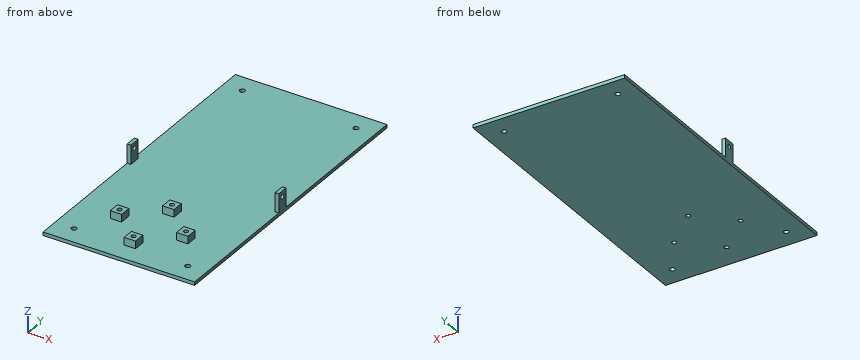
```python
from build123d import *

# Parameters (mm, degrees)
F0_R     = 7
F0_W     = 30
F0_H     = 30
F1_DEPTH = 9
F0_R_2   = 6
F2_DEPTH = 29
F0_W_2   = 10
F3_DEPTH = 59
F4_R     = 6
F5_DEPTH = 486


with BuildPart() as f1:
    # F0 (on Top) → F1 (new body)
    with BuildSketch(Plane.XY):
        Polygon((0, 350), (0, 0), (400, 0), (400, 350), (390, 350), (390, 380), (400, 380), (400, 800), (0, 800), (0, 380), (10, 380), (10, 350), align=None)
        with Locations((50, 50)):
            Circle(F0_R, mode=Mode.SUBTRACT)
        with Locations((197.5, 65)):
            Rectangle(F0_W, F0_H, mode=Mode.SUBTRACT)
        with Locations((110, 145)):
            Rectangle(F0_W, F0_H, mode=Mode.SUBTRACT)
        with Locations((197.5, 225)):
            Rectangle(F0_W, F0_H, mode=Mode.SUBTRACT)
        with Locations((285, 145)):
            Rectangle(F0_W, F0_H, mode=Mode.SUBTRACT)
        with Locations((350, 50)):
            Circle(F0_R, mode=Mode.SUBTRACT)
        with Locations((50, 750)):
            Circle(F0_R, mode=Mode.SUBTRACT)
        with Locations((350, 750)):
            Circle(F0_R, mode=Mode.SUBTRACT)
    extrude(amount=F1_DEPTH)

    # F0 (on Top) → F2 (join)
    with BuildSketch(Plane.XY):
        with Locations((110, 145)):
            Rectangle(F0_W, F0_H)
        with Locations((110, 145)):
            Circle(F0_R_2, mode=Mode.SUBTRACT)
        with Locations((197.5, 225)):
            Rectangle(F0_W, F0_H)
        with Locations((197.5, 225)):
            Circle(F0_R_2, mode=Mode.SUBTRACT)
        with Locations((197.5, 65)):
            Rectangle(F0_W, F0_H)
        with Locations((197.5, 65)):
            Circle(F0_R_2, mode=Mode.SUBTRACT)
        with Locations((285, 145)):
            Rectangle(F0_W, F0_H)
        with Locations((285, 145)):
            Circle(F0_R_2, mode=Mode.SUBTRACT)
    extrude(amount=F2_DEPTH)

    # F0 (on Top) → F3 (join)
    with BuildSketch(Plane.XY):
        with Locations((5, 365)):
            Rectangle(F0_W_2, F0_H)
        with Locations((395, 365)):
            Rectangle(F0_W_2, F0_H)
    extrude(amount=F3_DEPTH)

    # F4 (on Right) → F5 (cut)
    with BuildSketch(Plane.YZ):
        with Locations((365, 44)):
            Circle(F4_R)
    extrude(amount=F5_DEPTH, mode=Mode.SUBTRACT)


solid = f1.part
```
The listing builds one solid part. Answer for the finished solid, in the listing's coordinates (mm). Round coordinates to 2 decimals unless told otherwise and drop trailing zeros. Order: outer loops, then holes, each group sorted by start corner. A loop starts at its lowest first (then second) coordinate and runs counter-clockwise, first axis right, second up. Notation, with made-up numbers: (-35.5, -10) -> (-8.5, -10) arc R30 cw to (-8.5, 25) -> close; hole circle Ø9 at (-28, -37.75). An arc over 180 degrees is marked (long way). Answer as CSV lines item,"result". Start each with the question number.
(1) Flat-ended cylindrical pins translate along their axes: pin 1 Ø10 at (x, y) = (120.5, 543.5) entering from +Z; pin 2 Ø22 at (x, z) = (192.5, 18.5) entering from -Y; pin 3 Ø3 at (x, z) = (3, 29.5) entering from +Y; pin 4 Ø3 at (x, z) = (3, 37.5) entering from -Y. Find the tip coordinate at first contact, or state that the pin passes through.
(2) The part is cut by section A-A (y = 172). Determine the outline of the cut face in (x, z).
(3) The part is cut by section B-B (x = 260). Determine the outline of the cut face in (y, z), then the cut area to 3 significant figures.
(4) Find the intervals of material crossed by probe 1 along Y at (x, z) = (197, 10); probe 2 along X at (y, z) = (750, 5.5); probe 3 along Y at (x, z) = (284.5, 14), in increasing order. Write a range as from..to.
Evaluation:
1,pin 1,"z = 9"
1,pin 2,"y = 0"
1,pin 3,"y = 380"
1,pin 4,"y = 350"
2,outline,"(0, 0) -> (400, 0) -> (400, 9) -> (0, 9) -> close"
3,outline,"(0, 0) -> (800, 0) -> (800, 9) -> (0, 9) -> close"
3,area,"7,200 mm²"
4,probe 1,"50..59.02, 70.98..80, 210..219.02, 230.98..240"
4,probe 2,"0..43, 57..343, 357..400"
4,probe 3,"130..139.02, 150.98..160"
